from build123d import *

# Parameters (mm, degrees)
BOSS_EXTRUDE1_DEPTH = 12
SKETCH3_R           = 20
SKETCH3_R_2         = 10
BOSS_EXTRUDE2_DEPTH = 30
BOSS_EXTRUDE3_DEPTH = 10
SKETCH5_R           = 5.5
CUT_EXTRUDE1_DEPTH  = 97.587759017
SKETCH6_W           = 8
SKETCH6_H           = 4
BOSS_EXTRUDE4_DEPTH = 85
SKETCH7_W           = 5
SKETCH7_H           = 20.431914742
BOSS_EXTRUDE5_DEPTH = 15


with BuildPart() as part:
    # Sketch2 → Boss-Extrude1 (new body)
    with BuildSketch(Plane(origin=(0, 0, 0), x_dir=(1, 0, 0), z_dir=(0, 1, 0))):
        with BuildLine():
            Line((-18.765432099, -74.580246914), (-18.765432099, 10.419753086))
            Line((-18.765432099, 10.419753086), (24.234567901, 10.419753086))
            ThreePointArc((24.234567901, 10.419753086), (27.770101807, 8.955286992), (29.234567901, 5.419753086))
            Line((29.234567901, 5.419753086), (29.234567901, -69.580246914))
            ThreePointArc((29.234567901, -69.580246914), (27.770101807, -73.11578082), (24.234567901, -74.580246914))
            Line((24.234567901, -74.580246914), (-18.765432099, -74.580246914))
        make_face()
    extrude(amount=-BOSS_EXTRUDE1_DEPTH)



with BuildPart() as body_2:
    # Sketch3 → Boss-Extrude2 (new body)
    with BuildSketch(Plane.ZY.offset(18.765432099)):
        with Locations((32.080246914, 33.965933716)):
            Circle(SKETCH3_R)
        with Locations((32.080246914, 33.965933716)):
            Circle(SKETCH3_R_2, mode=Mode.SUBTRACT)
    extrude(amount=-BOSS_EXTRUDE2_DEPTH)


with BuildPart() as part_1:
    add(part.part)

    add(body_2.part)  # Boss-Extrude3 merges body 2
    # Sketch4 → Boss-Extrude3 (add)
    with BuildSketch(Plane.ZY.offset(18.765432099)):
        with BuildLine():
            Line((12.080246914, 33.965933716), (-10.419753086, 0))
            Line((-10.419753086, 0), (74.580246914, 0))
            Line((74.580246914, 0), (52.080246914, 33.965933716))
            ThreePointArc((52.080246914, 33.965933716), (32.080246914, 13.965933716), (12.080246914, 33.965933716))
        make_face()
    extrude(amount=-BOSS_EXTRUDE3_DEPTH)

    # Sketch5 → Cut-Extrude1 (cut, through all)
    with BuildSketch(Plane(origin=(0, 0, 0), x_dir=(1, 0, 0), z_dir=(0, 1, 0))):
        with Locations(Location((11.234567901, -2.080246914, 0), (0, 0, 270))):
            Circle(SKETCH5_R)
        with Locations(Location((11.234567901, -62.080246914, 0), (0, 0, 270))):
            Circle(SKETCH5_R)
    extrude(amount=-CUT_EXTRUDE1_DEPTH, mode=Mode.SUBTRACT)

    # Sketch6 → Boss-Extrude4 (add)
    with BuildSketch(Plane.XY.offset(74.580246914)):
        with Locations((-14.765432099, -14)):
            Rectangle(SKETCH6_W, SKETCH6_H)
    extrude(amount=-BOSS_EXTRUDE4_DEPTH)

    # Sketch7 → Boss-Extrude5 (add)
    with BuildSketch(Plane.ZY.offset(8.765432099)):
        Polygon((36.436270076, 20.431914742), (31.436270076, 20.431914742), (31.436270076, 0), (36.436270076, 0), (36.436270076, 14.206805316), align=None)
        with Locations((28.936270076, 10.215957371)):
            Rectangle(SKETCH7_W, SKETCH7_H)
    extrude(amount=-BOSS_EXTRUDE5_DEPTH)


solid = part_1.part
For this review, take the finished solid that the model builds, in its own axes (mm). A direction names the side the tool comes from. Round coordinates to 2 decimals unless told otherwise and drop trailing zeros. Loops run counter-clockwise (first coordinate to the right, second up) from the corner with the lowest first, then second, coordinate; pieces in that order, holes last. Notation, with made-up numbers: (-37.5, 17.5) - (-25.5, 17.5) arc R15 cw to (-25.5, 37.5) - close; hole circle Ø9 at (25, -10). An arc over 180 degrees is marked (long way). Use one line per item in the form item = value.
Item 1: Tool access review of faces 1 (the flat face through (10, -12, 31)), 2 (the flat face through (-8.765, 10, 55)), 3 (the flat face through (11.235, 43, 27)), 4 (the flat face through (-8.765, 13, 12)): name each direction out of +Z, -Z, +X, -X, +Y, -Y from which nothing blocks a thin tool from reaching the whole face with its end or side.
Answers:
face_1 = +Z, -Z, +X, -Y
face_2 = +Z, +X
face_3 = +Z, -Z, +X, +Y
face_4 = -Z, +X
Item 2: Mouldability with a two-part tool opening along Y and no side actions: class faces 5 (the flat face through (-15, -16, 33)), 6 (the flat face through (11, 0, 31)), 7 (the cylindrical face through (27.809, -5.916, 73.077)) as +Y half, -Y half, draft (parallel to the pull), parting line (faces both ways), or undercut.
Answers:
face_5 = -Y half
face_6 = undercut
face_7 = draft
Item 3: Consider section C-C on z = 24. Write out the cut boundary in (x, y), then the cut area to 3 significant figures.
Answers:
outline = (-18.77, -16) - (-10.77, -16) - (-10.77, -12) - (29.23, -12) - (29.23, 0) - (-8.77, 0) - (-8.77, 15.67) - (11.23, 15.67) - (11.23, 28.07) - (-18.77, 28.07) - close; (-18.77, 39.86) - (11.23, 39.86) - (11.23, 52.26) - (-18.77, 52.26) - close
area = 1,510 mm^2
Item 4: For line 1 (Y direction, x = -1, z = 59); line 2 (X direction, y = 6, z = -4); line 3 (Z direction, x = -4, y = 36.5), list the stretches that pass through material, from the lowest coordinate up.
Answers:
line_1 = -12 to 0
line_2 = -18.77 to -8.77
line_3 = 12.24 to 22.41, 41.75 to 51.92
Item 5: Consider section B-B on x = -14. Write out the cut boundary in (y, z), then the cut area to 3 significant figures.
Answers:
outline = (-16, -10.42) - (0, -10.42) - (33.97, 12.08) arc R20 ccw to (33.97, 52.08) - (0, 74.58) - (-16, 74.58) - close; hole circle Ø20 at (33.97, 32.08)
area = 3,800 mm^2
Item 6: Clearance check with flat-ended pins moving along their axes: P1, Ø11, axis at y = 5, z = 30, coming from the +X side; P2, Ø12, axis at y = 9.5, z = 43.5, coming from the +X side; P3, Ø10, axis at y = 25, z = 52, coming from the +X side; P4, Ø6, axis at x = 3.5, z = 9.5, coming from the -Y side. State where each tip first meets the part, or that it passes through.
Answers:
P1 = 29.23
P2 = -8.77
P3 = 11.23
P4 = -12
Item 7: Consider section A-A on y = -8. Write out the cut boundary in (x, z), then the cut area to 3 significant figures.
Answers:
outline = (-18.77, -10.42) - (24.23, -10.42) arc R5 ccw to (29.23, -5.42) - (29.23, 69.58) arc R5 ccw to (24.23, 74.58) - (-18.77, 74.58) - close; hole circle Ø11 at (11.23, 2.08); hole circle Ø11 at (11.23, 62.08)
area = 3,880 mm^2
Item 8: Consider section D-D on x = 13.5. Write out the cut boundary in (y, z), then the cut area to 3 significant figures.
Answers:
outline = (-12, -10.42) - (0, -10.42) - (0, -2.93) - (-12, -2.93) - close; (-12, 7.09) - (0, 7.09) - (0, 57.07) - (-12, 57.07) - close; (-12, 67.09) - (0, 67.09) - (0, 74.58) - (-12, 74.58) - close
area = 779 mm^2
